Input: part model. Units: mm. Frame: model coordinates. Give positions to 0.01 mm unless a question says otherwise; leave off trailing zeros. Loops run counter-clockwise (first coordinate to the right, second up) from the corner with the lowest first, then second, coordinate; pieces in that order, holes last. Notation, with made-up numbers: (4.25, -36.75) - (30.25, -36.75) arc R28 cw to (30.25, -6.75) - close; hole circle Ø9 at (-36.75, 54.25). An arc over 180 degrees is marked (long way). One line per item, written item: value.
Autodesk Inventor part; units mm, degrees
ref_plane "YZ Plane" through (0, 0, 0) normal (1, 0, 0) x (0, 1, 0)
ref_plane "XZ Plane" through (0, 0, 0) normal (0, 1, 0) x (-1, 0, 0)
ref_plane "XY Plane" through (0, 0, 0) normal (0, 0, 1) x (1, 0, 0)
sketch "Sketch1" plane through (0, 0, 0) normal (0, 0, 1) x (1, 0, 0)
  line L0 (0, 0) -> (135.404, 0) construction
  line L1 (0, -4.8511) -> (135.404, -4.8511)
  line L2 (135.404, 4.8511) -> (0, 4.8511)
  arc A0 (0, 4.8511) -> (0, -4.8511) centre (0, 0) ccw
  arc A1 (135.404, -4.8511) -> (135.404, 4.8511) centre (135.404, 0) ccw
  circle A2 centre (0, 0) radius 2.125
  circle A3 centre (135.404, 0) radius 2.125
  point P0 (67.702, 0)
  point P1 (0.702, -2.0057)
  point P2 (0.702, 2.0057)
  dimension "d0" = 135.404
  dimension "d1" = 4.25
extrude "Extrusion1" add sketch "Sketch1" along normal blind 3
properties part number "linkage"
Item 1: Section B-B, the plane z = 0.95. Output: boundary loops of the cut face in (x, y) (3 decimals).
Verdict:
outline: (0, -4.851) - (135.404, -4.851) arc R4.851 ccw to (135.404, 4.851) - (0, 4.851) arc R4.851 ccw to start; hole circle Ø4.25 at (0, 0); hole circle Ø4.25 at (135.404, 0)
Item 2: Material intervals for L1, parallel to Y at x = 0, z = 1.3 (3 decimals); L2, parallel to X at y = -0.25, z = 1; L3, parallel to X at y = -1, z = 1.4 (3 decimals), sorted ascending.
Verdict:
L1: y = -4.851 to -2.125, 2.125 to 4.851
L2: x = -4.84 to -2.11, 2.11 to 133.29, 137.51 to 140.25
L3: x = -4.747 to -1.875, 1.875 to 133.529, 137.279 to 140.151
Item 3: Draft query along Y for faces 1 (the face through (69, 4.851, 1)), 2 (the face through (140.254, 0.107, 1.479)), 3 (the face through (1.142, -1.792, 1.479)). Return one class per face: pulls with the +Y half, pulls with the -Y half, needs draft (parallel to the pull), parting line crosses it, or undercut.
Verdict:
face 1: pulls with the +Y half
face 2: parting line crosses it
face 3: undercut
Item 4: Pin query (flat end, axial travel): P1, Ø1.5, axis at y = -1.5, z = 1, coming from the -X side; P2, Ø1.5, axis at y = 3.5, z = 0.5, coming from the +X side. Return the tip coordinate at first contact, or that it passes through.
Verdict:
P1: stops at x = -4.79
P2: stops at x = 139.4
Item 5: Section A-A, the plane y = 0. Output: boundary loops of the cut face in (x, z) (3 decimals).
Verdict:
outline: (-4.851, 0) - (-2.125, 0) - (-2.125, 3) - (-4.851, 3) - close; (2.125, 0) - (133.279, 0) - (133.279, 3) - (2.125, 3) - close; (137.529, 0) - (140.255, 0) - (140.255, 3) - (137.529, 3) - close
